Can you work these out from the drawing? Everything is in mm from the part's minimum corner. A direction names the side the tool comes from. Coordinates: 2 decimals unless noted, no trailing zeros. Order: outer loops, then holes, each group sorted by start corner. A loop starts at its lowest first (then second) coordinate and runs counter-clockwise, first axis right, second up. Notation, with made-up numbers: M 45,41.5 L 65,41.5 A11 ccw 65,59.5 Z; hole C 72,49.5 d10. An arc over 180 degrees is marked long. Answer as a JSON object with one key per item and string values.
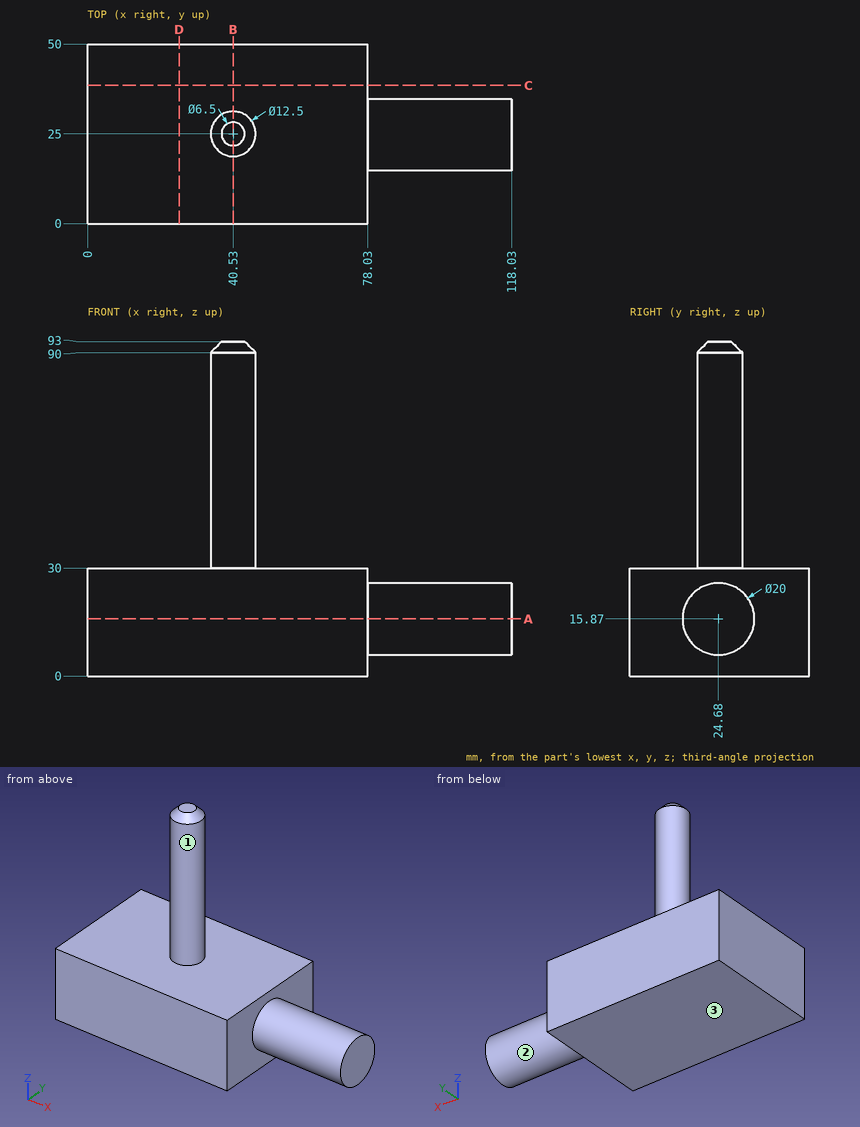
Item 1: I want a section at C-C, the plane y = 38.5. Write out the boundary of the cut face in (x, z), plus the area to 3 significant figures.
Answers follow:
{"outline": "M 0,0 L 78.03,0 L 78.03,30 L 0,30 Z", "area": "2,340 mm^2"}
Item 2: I want a section at D-D, the plane x = 25.5. Write out the boundary of the cut face in (y, z).
Answers follow:
{"outline": "M 0,0 L 50,0 L 50,30 L 0,30 Z"}
Item 3: Please list where these lines run through material, in increasing order: line 1 (Z direction, x = 14, y = 17); line 2 (X direction, y = 4.5, z = 9); line 3 (X direction, y = 21.5, z = 83.5).
Answers follow:
{"line 1": "z = 0 to 30", "line 2": "x = 0 to 78.03", "line 3": "x = 35.35 to 45.71"}
Item 4: I want a section at B-B, the plane x = 40.53. Write out the boundary of the cut face in (y, z).
Answers follow:
{"outline": "M 0,0 L 50,0 L 50,30 L 31.25,30 L 31.25,90 L 28.25,93 L 21.75,93 L 18.75,90 L 18.75,30 L 0,30 Z"}
Item 5: I'm going to push flat-ended pins straight in: pin 1 (2 mm diameter, centred on x = 81.5, y = 15, fed in from -Z); pin 2 (12 mm diameter, centred on x = 13.5, y = 17.5, fed in from +Z); pin 3 (1 mm diameter, centred on y = 29, z = 42, fed in from -X); pin 4 (1 mm diameter, centred on x = 48, z = 61.5, fed in from -Y). Where does each tip first touch, or does it pass through?
Answers follow:
{"pin 1": "stops at z = 10.9", "pin 2": "stops at z = 30", "pin 3": "stops at x = 35.35", "pin 4": "passes through"}
Item 6: Which directions (+Z, -Z, +X, -X, +Y, -Y) give clear straight access to the entire face, cutting with the end or side of a thin tool? Please do the marked faces 1, 2 and 3.
Answers follow:
{"face 1": "+Z", "face 2": "+X", "face 3": "-Z, +X, -X, +Y, -Y"}
Item 7: I want a section at A-A, the plane z = 15.87. Write out the boundary of the cut face in (x, y).
Answers follow:
{"outline": "M 0,0 L 78.03,0 L 78.03,14.68 L 118.03,14.68 L 118.03,34.68 L 78.03,34.68 L 78.03,50 L 0,50 Z"}
